from build123d import *

# Parameters (mm, degrees)
F0_W      = 40
F0_H      = 120
F1_DEPTH  = 40
F2_W      = 10
F2_H      = 40
F3_DEPTH  = 40
F4_W      = 10
F4_H      = 40
F5_DEPTH  = 40
F6_W      = 10
F6_H      = 40
F7_DEPTH  = 40
F8_R      = 10
F9_DEPTH  = 25
F10_R     = 10
F11_DEPTH = 25
F12_R     = 19.99999


# Not quite as in the source:
# - a fillet or chamfer is up to 0.001 mm smaller than in the source, because OpenCascade refuses the exact size


with BuildPart() as f1:
    # F0 (on Front) → F1 (new body)
    with BuildSketch(Plane.XZ):
        Rectangle(F0_W, F0_H)
    extrude(amount=F1_DEPTH)

    # F2 (on face) → F3 (cut)
    with BuildSketch(Plane.XZ.offset(40)):
        with Locations((-15, 40)):
            Rectangle(F2_W, F2_H)
    extrude(amount=-F3_DEPTH, mode=Mode.SUBTRACT)

    # F4 (on face) → F5 (cut)
    with BuildSketch(Plane.XZ.offset(40)):
        with Locations((15, 40)):
            Rectangle(F4_W, F4_H)
    extrude(amount=-F5_DEPTH, mode=Mode.SUBTRACT)

    # F6 (on face) → F7 (cut)
    with BuildSketch(Plane.XZ.offset(40)):
        with Locations((-15, -40)):
            Rectangle(F6_W, F6_H)
        with Locations((15, -40)):
            Rectangle(F6_W, F6_H)
    extrude(amount=-F7_DEPTH, mode=Mode.SUBTRACT)

    # F8 (on face) → F9 (cut)
    with BuildSketch(Plane.YZ.offset(10)):
        with Locations((-20, 40)):
            Circle(F8_R)
    extrude(amount=-F9_DEPTH, mode=Mode.SUBTRACT)

    # F10 (on face) → F11 (cut)
    with BuildSketch(Plane.YZ.offset(10)):
        with Locations((-20, -40)):
            Circle(F10_R)
    extrude(amount=-F11_DEPTH, mode=Mode.SUBTRACT)

    # F12 (radius 20 in the source; OpenCascade refuses exactly that, so slightly less here)
    f12_edges = [f1.edges().sort_by_distance(p)[0] for p in [
        (0, -40, 60),
        (0, 0, 60),
        (0, -40, -60),
        (0, 0, -60),
    ]]
    fillet(f12_edges, radius=F12_R)


solid = f1.part
Geometry: final body of the model. Coordinates: model frame, mm. A direction names the side the tool comes from. Round coordinates to 2 decimals unless told otherwise and drop trailing zeros. Loops run counter-clockwise (first coordinate to the right, second up) from the corner with the lowest first, then second, coordinate; pieces in that order, holes last.
Q1. Material intervals for L1, parallel to Z at x = 1, y = -20; L2, parallel to Z at x = 0, y = -14.5; L3, parallel to X at y = -16, z = 20.5, sorted ascending.
Q2. Pull-direction query (Z, two-part tool) for faces 5 (the cylindrical face through (0.14, -15.386, -48.872)), 6 (the cylindrical face through (0.14, -15.386, 31.128)), 7 (the cylindrical face through (0.14, -34.297, 53.986)), 8 (the flat face through (0, 0, 1)); classes: released by +Z, released by -Z, zero draft, split by the parting line, or undercut.
Q3. Section C-C on z = 44. Return loops of the section in (x, y), plus the area to 3 significant figures.
Q4. Pin query (flat end, axial travel): P1, Ø3, axis at x = -17.5, y = -29, coming from the +Z side; P2, Ø5, axis at x = 3.5, y = -31, coming from the +Z side; P3, Ø12, axis at x = -7, y = -12.5, coming from the -Z side; P4, Ø12, axis at y = -18.5, z = 40, coming from the +X side. Return the tip coordinate at first contact, or that it passes through.
Q5. Access query for faces 1 (the flat face through (-10, -20, -27)), 2 (the flat face through (-15, -20, 20)), 3 (the flat face through (10, -25, 31)), 4 (the flat face through (15, -20, -20)). Directions: +Z, -Z, +X, -X, +Y, -Y. A direction counts if a zero-diameter tool reaches every point of the face in a straight line with its end or side. Return the directions, or none.
Q6. Section A-A on x = 8. State how many separate pieces and enclosed holes the cut face has, plus the area to 3 significant figures.
Q7. Section D-D on x = 15. Return loops of the section in (y, z), plus the area to 3 significant figures.
Q8. Section B-B on y = -14. Return loops of the section in (x, z).
Evaluation:
1. L1: z = -60 to -50, -30 to 30, 50 to 60
1. L2: z = -59.23 to -48.35, -31.65 to 31.65, 48.35 to 59.23
1. L3: x = -10 to 10
2. face 5: undercut
2. face 6: undercut
2. face 7: released by +Z
2. face 8: zero draft
3. outline: (-10, -39.6) - (10, -39.6) - (10, -29.17) - (-10, -29.17) - close; (-10, -10.83) - (10, -10.83) - (10, -0.4) - (-10, -0.4) - close
3. area: 417 mm2
4. P1: stops at z = 20
4. P2: stops at z = 58.1
4. P3: stops at z = -59.94
4. P4: passes through
5. face 1: -Z, -X, +Y, -Y
5. face 2: +Z, -X, +Y, -Y
5. face 3: +Z, +X, +Y, -Y
5. face 4: -Z, +X, +Y, -Y
6. separate pieces: 1
6. enclosed holes: 2
6. area: 3,830 mm2
7. outline: (-40, -20) - (0, -20) - (0, 20) - (-40, 20) - close
7. area: 1,600 mm2
8. outline: (-20, -20) - (-10, -20) - (-10, -32) - (10, -32) - (10, -20) - (20, -20) - (20, 20) - (10, 20) - (10, 32) - (-10, 32) - (-10, 20) - (-20, 20) - close; (-10, -59.08) - (10, -59.08) - (10, -48) - (-10, -48) - close; (-10, 48) - (10, 48) - (10, 59.08) - (-10, 59.08) - close
